from build123d import *

# Parameters (mm, degrees)
F1_DEPTH = 8
F2_R     = 0.99999
F3_R     = 0.5


# Not quite as in the source:
# - a fillet or chamfer is up to 0.001 mm smaller than in the source, because OpenCascade refuses the exact size


with BuildPart() as f1:
    # F0 (on Front) → F1 (new body)
    with BuildSketch(Plane.XZ):
        Polygon((1.5, -2.5), (1.5, 2.5), (0.5, 2.5), (0.5, -1.5), (-0.5, -1.5), (-0.5, 2.5), (-1.5, 2.5), (-1.5, -2.5), align=None)
    extrude(amount=F1_DEPTH)

    # F2 (radius 1 in the source; OpenCascade refuses exactly that, so slightly less here)
    f2_edges = [f1.edges().sort_by_distance(p)[0] for p in [
        (0, -8, -2.5),
    ]]
    fillet(f2_edges, radius=F2_R)

    # F3
    f3_edges = [f1.edges().sort_by_distance(p)[0] for p in [
        (-1.5, -3.500005, -2.5),
        (1.5, -3.500005, -2.5),
        (1.5, -4, 2.5),
        (-1.5, -4, 2.5),
        (-1, -8, 2.5),
        (1, -8, 2.5),
    ]]
    fillet(f3_edges, radius=F3_R)


solid = f1.part
Verification items for the finished model (mm, model axes). A direction names the side the tool comes from. Coordinates: 2 decimals unless noted, no trailing zeros. Write each loop counter-clockwise with the first axis right and the second up, starting at its lowest first coordinate (ties: lowest second). Pieces come first, ordered by that corner, then holes. Notation, with made-up numbers: (48, 4.25) -> (66, 4.25) arc R25 ccw to (66, 24.25) -> close; hole circle Ø6 at (57.25, -3.75). An arc over 180 degrees is marked (long way). One line per item, written item: value. Start each with the question number.
Q1. Cross-section at A-A on z = 1.1. Enter the section's corners in (x, y), and give its area (3 significant figures).
Q2. Mould release check, pull along X, two halves, no side actions. Record for faces 1 (the flat face through (0, -4, -1.5)), 2 (the flat face through (1.5, -4, 0)), 3 (the flat face through (-1.5, -4, 0)): pulls with the +X half, pulls with the -X half, needs draft (parallel to the pull), parting line crosses it, or undercut.
Q3. Access from +Z, -Z, +X, -X, +Y, -Y to the whole of each face (thin tool, end or side, straight path). Record for faces 4 (the flat face through (0.5, -4, 1)), 5 (the cylindrical face through (0.014, -7.699, -2.215)).
Q4. Go/stop test with a flat-tipped pin: P1, Ø0.5, axis at x = 0, y = -4, coming from the +Z side. Record where the tip stops, or that it passes through.
Q5. Cross-section at B-B on y = -5. Enter the section's corners in (x, z), and give its area (3 significant figures).
Q6. Thickness scan on L1, parallel to X at y = -7.5, z = -0.65; L2, parallel to Y at x = 1.05, z = 1.9; L3, parallel to X at y = -6.25, z = 2.3. Record the ranges inside material, lowest first. Write a range as from..to.
Checked values:
1. outline: (-1.5, -7.5) arc R0.5 ccw to (-1, -8) -> (-0.5, -8) -> (-0.5, 0) -> (-1.5, 0) -> close; (0.5, -8) -> (1, -8) arc R0.5 ccw to (1.5, -7.5) -> (1.5, 0) -> (0.5, 0) -> close
1. area: 15.9 mm²
2. face 1: undercut
2. face 2: pulls with the +X half
2. face 3: pulls with the -X half
3. face 4: +Z, +Y, -Y
3. face 5: -Z, +X, -X, -Y
4. P1: stops at z = -1.5
5. outline: (-1.5, -2) arc R0.5 ccw to (-1, -2.5) -> (1, -2.5) arc R0.5 ccw to (1.5, -2) -> (1.5, 2) arc R0.5 ccw to (1, 2.5) -> (0.5, 2.5) -> (0.5, -1.5) -> (-0.5, -1.5) -> (-0.5, 2.5) -> (-1, 2.5) arc R0.5 ccw to (-1.5, 2) -> close
5. area: 10.8 mm²
6. L1: x = -1.5..-0.5, 0.5..1.5
6. L2: y = -8..0
6. L3: x = -1.4..-0.5, 0.5..1.4
